Can you work these out from the model? Positions are in its coordinate system, mm. Face numbers are marked on the shaded views. A direction names the side the tool comes from. Coordinates: 2 decimals unless noted, no trailing zeros. Order: outer loops, then holes, each group sorted by start corner. A loop starts at its lowest first (then second) coordinate and runs counter-clockwise, first axis right, second up. Notation, with made-up numbers: (31, -7) -> (40, -7) arc R17 cw to (40, 25) -> close; hole circle Ø6 at (45, -19.5). An arc over 180 degrees is marked (long way). Return JSON: item names as keys, results as strings. Group by question number.
1) If we section it at A-A, the plane y = -1.5: Please give me the cut outline in (x, z), then the cut area to 3 significant figures.
2) If we section it at B-B, the plane z = 7: State how many separate pieces and enclosed holes the cut face has, then the cut area to 3 significant figures.
3) If we section it at C-C, the plane x = -0.25: Please give me the cut outline in (y, z), then the cut area to 3 significant figures.
4) If I drill on probe 1 along Y at (x, z) = (0, 5.75); probe 2 along Y at (x, z) = (-0.25, 4); probe 3 along X at (y, z) = (2.5, 6.5), over which ranges is the centre line in solid material (lowest first)? Write a range as from..to.
5) Thinking about a two-plate mould opening in X: for the marked faces 1, 2 and 3, which applies, +X half, -X half, draft (parallel to the pull), parting line (faces both ways), or undercut?
6) For the marked faces 4 and 5, which set-ups out of +Z, -Z, +X, -X, +Y, -Y let a thin tool reach every point of the face, with its end or its side?
7) If we section it at D-D, the plane x = -1.75: Please give me the cut outline in (y, z).
8) For pin 1 (0.7 mm diameter, centred on y = 7.5, z = 0.5, fed in from +X); pin 2 (1.3 mm diameter, centred on x = 2, z = 3, fed in from -Y); pin 3 (1.3 mm diameter, centred on x = -2, z = 4, fed in from +Y); pin 4 (1.2 mm diameter, centred on x = 0, y = -5.8, fed in from -Z), each with a flat end and sliding along its axis, tell me the tip position at first contact or that it passes through.
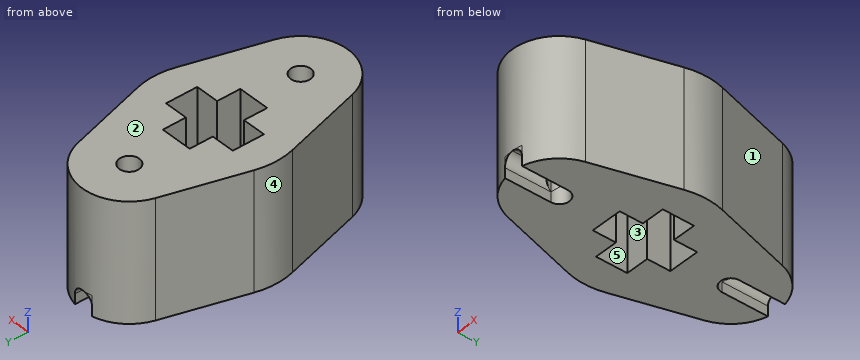
from build123d import *

# Parameters (mm, degrees)
F0_R         = 0.6731
F1_DEPTH     = 7.9375
F3_DEPTH     = 1.3462
F4_T4_DEPTH  = 6.4683311894
F4_S5_R      = 3.175
F4_T6_DEPTH  = 5
F4_S7_R      = 0.6731
F4_T8_DEPTH  = 5
F4_T12_DEPTH = 6.4683311894
F4_S13_R     = 3.175
F4_T14_DEPTH = 5
F4_S15_R     = 0.6731
F4_T16_DEPTH = 5
F4_T20_DEPTH = 6.4683311894
F4_S21_R     = 3.175
F4_T22_DEPTH = 5
F4_S23_R     = 0.6731
F4_T24_DEPTH = 5
F4_T28_DEPTH = 6.4683311894
F4_S29_R     = 3.175
F4_T30_DEPTH = 5
F4_S31_R     = 0.6731
F4_T32_DEPTH = 5


# Not quite as in the source:
# - a fillet or chamfer that OpenCascade refuses, or shapes differently, is made with other operations: its cross-section is extruded or revolved along the edge and cut away or added


with BuildPart() as f1:
    # F0 (on Top) → F1 (new body)
    with BuildSketch(Plane.XY):
        with BuildLine():
            ThreePointArc((-4.5806904159, 1.3033347856), (-4.7625, 0), (-4.5806904159, -1.3033347856))
            Line((-4.5806904159, -1.3033347856), (-3.0537936106, -6.6697545571))
            ThreePointArc((-3.0537936106, -6.6697545571), (0, -8.9758647), (3.0537936106, -6.6697545571))
            Line((3.0537936106, -6.6697545571), (4.5806904159, -1.3033347856))
            ThreePointArc((4.5806904159, -1.3033347856), (4.7625, 0), (4.5806904159, 1.3033347856))
            Line((4.5806904159, 1.3033347856), (3.0537936106, 6.6697545571))
            ThreePointArc((3.0537936106, 6.6697545571), (0, 8.9758647), (-3.0537936106, 6.6697545571))
            Line((-3.0537936106, 6.6697545571), (-4.5806904159, 1.3033347856))
        make_face()
        with Locations((0, -5.8008647)):
            Circle(F0_R, mode=Mode.SUBTRACT)
        Polygon((-1.0574147, 2.6258647), (1.0574147, 2.6258647), (1.0574147, 1.0574147), (2.6258647, 1.0574147), (2.6258647, -1.0574147), (1.0574147, -1.0574147), (1.0574147, -2.6258647), (-1.0574147, -2.6258647), (-1.0574147, -1.0574147), (-2.6258647, -1.0574147), (-2.6258647, 1.0574147), (-1.0574147, 1.0574147), align=None, mode=Mode.SUBTRACT)
        with Locations((0, 5.8008647)):
            Circle(F0_R, mode=Mode.SUBTRACT)
    extrude(amount=F1_DEPTH)

    # F2 (on face) → F3 (cut)
    with BuildSketch(Plane(origin=(0, 0, 0), x_dir=(1, 0, 0), z_dir=(0, 0, -1))):
        with BuildLine():
            Line((-0.6731, 5.8008647), (0.6731, 5.8008647))
            Line((0.6731, 5.8008647), (0.6731, 8.9036958894))
            ThreePointArc((0.6731, 8.9036958894), (0, 8.9758647), (-0.6731, 8.9036958894))
            Line((-0.6731, 8.9036958894), (-0.6731, 5.8008647))
        make_face()
        with BuildLine():
            Line((0.6731, -8.9036958894), (0.6731, -5.8008647))
            Line((0.6731, -5.8008647), (-0.6731, -5.8008647))
            Line((-0.6731, -5.8008647), (-0.6731, -8.9036958894))
            ThreePointArc((-0.6731, -8.9036958894), (0, -8.9758647), (0.6731, -8.9036958894))
        make_face()
    extrude(amount=-F3_DEPTH, mode=Mode.SUBTRACT)

    # F4: fillet of radius 0.6731 on 4 edges, made by hand


with BuildPart() as f4_tool2:
    # F4_s3 → F4_t4 (new body)
    with BuildSketch(Plane.XZ.offset(-10.5864458894)):
        with BuildLine():
            ThreePointArc((0.6731, 0.6731), (0.4759535744, 1.1490535744), (0, 1.3462))
            Line((0, 1.3462), (0.6731, 1.3462))
            Line((0.6731, 1.3462), (0.6731, 0.6731))
        make_face()
    extrude(amount=F4_T4_DEPTH)

    # F4_s5 → F4_t6 (intersect, symmetric)
    with BuildSketch(Plane.XY.offset(1)):
        with Locations((0, 5.8008647)):
            Circle(F4_S5_R)
    extrude(amount=F4_T6_DEPTH, both=True, mode=Mode.INTERSECT)

    # F4_s7 → F4_t8 (cut, symmetric)
    with BuildSketch(Plane.XY.offset(1)):
        with Locations((0, 5.8008647)):
            Circle(F4_S7_R)
    extrude(amount=F4_T8_DEPTH, both=True, mode=Mode.SUBTRACT)


with BuildPart() as f1_1:
    add(f1.part)

    # F4_t1: union F4_tool2
    add(f4_tool2.part)


with BuildPart() as f4_tool10:
    # F4_s11 → F4_t12 (new body)
    with BuildSketch(Plane.XZ.offset(-4.1181147)):
        with BuildLine():
            ThreePointArc((-0.6731, 0.6731), (-0.4759535744, 1.1490535744), (0, 1.3462))
            Line((0, 1.3462), (-0.6731, 1.3462))
            Line((-0.6731, 1.3462), (-0.6731, 0.6731))
        make_face()
    extrude(amount=-F4_T12_DEPTH)

    # F4_s13 → F4_t14 (intersect, symmetric)
    with BuildSketch(Plane.XY.offset(1)):
        with Locations((0, 5.8008647)):
            Circle(F4_S13_R)
    extrude(amount=F4_T14_DEPTH, both=True, mode=Mode.INTERSECT)

    # F4_s15 → F4_t16 (cut, symmetric)
    with BuildSketch(Plane.XY.offset(1)):
        with Locations((0, 5.8008647)):
            Circle(F4_S15_R)
    extrude(amount=F4_T16_DEPTH, both=True, mode=Mode.SUBTRACT)


with BuildPart() as f1_2:
    add(f1_1.part)

    # F4_t9: union F4_tool10
    add(f4_tool10.part)


with BuildPart() as f4_tool18:
    # F4_s19 → F4_t20 (new body)
    with BuildSketch(Plane.XZ.offset(4.1181147)):
        with BuildLine():
            ThreePointArc((0.6731, 0.6731), (0.4759535744, 1.1490535744), (0, 1.3462))
            Line((0, 1.3462), (0.6731, 1.3462))
            Line((0.6731, 1.3462), (0.6731, 0.6731))
        make_face()
    extrude(amount=F4_T20_DEPTH)

    # F4_s21 → F4_t22 (intersect, symmetric)
    with BuildSketch(Plane.XY.offset(1)):
        with Locations((0, -5.8008647)):
            Circle(F4_S21_R)
    extrude(amount=F4_T22_DEPTH, both=True, mode=Mode.INTERSECT)

    # F4_s23 → F4_t24 (cut, symmetric)
    with BuildSketch(Plane.XY.offset(1)):
        with Locations((0, -5.8008647)):
            Circle(F4_S23_R)
    extrude(amount=F4_T24_DEPTH, both=True, mode=Mode.SUBTRACT)


with BuildPart() as f1_3:
    add(f1_2.part)

    # F4_t17: union F4_tool18
    add(f4_tool18.part)


with BuildPart() as f4_tool26:
    # F4_s27 → F4_t28 (new body)
    with BuildSketch(Plane.XZ.offset(10.5864458894)):
        with BuildLine():
            ThreePointArc((-0.6731, 0.6731), (-0.4759535744, 1.1490535744), (0, 1.3462))
            Line((0, 1.3462), (-0.6731, 1.3462))
            Line((-0.6731, 1.3462), (-0.6731, 0.6731))
        make_face()
    extrude(amount=-F4_T28_DEPTH)

    # F4_s29 → F4_t30 (intersect, symmetric)
    with BuildSketch(Plane.XY.offset(1)):
        with Locations((0, -5.8008647)):
            Circle(F4_S29_R)
    extrude(amount=F4_T30_DEPTH, both=True, mode=Mode.INTERSECT)

    # F4_s31 → F4_t32 (cut, symmetric)
    with BuildSketch(Plane.XY.offset(1)):
        with Locations((0, -5.8008647)):
            Circle(F4_S31_R)
    extrude(amount=F4_T32_DEPTH, both=True, mode=Mode.SUBTRACT)


with BuildPart() as f1_4:
    add(f1_3.part)

    # F4_t25: union F4_tool26
    add(f4_tool26.part)


solid = f1_4.part
Result sheet:
{
 "1": {"outline": "(-4.52, 0) -> (-1.06, 0) -> (-1.06, 7.94) -> (-4.52, 7.94) -> close; (1.06, 0) -> (4.52, 0) -> (4.52, 7.94) -> (1.06, 7.94) -> close", "area": "55.0 mm2"},
 "2": {"separate pieces": "1", "enclosed holes": "3", "area": "107 mm2"},
 "3": {"outline": "(-8.97, 1.3) -> (-6.43, 1.3) -> (-6.43, 7.94) -> (-8.97, 7.94) -> close; (-5.18, 0) -> (-2.63, 0) -> (-2.63, 7.94) -> (-5.18, 7.94) -> close; (2.63, 0) -> (5.18, 0) -> (5.18, 7.94) -> (2.63, 7.94) -> close; (6.43, 1.3) -> (8.97, 1.3) -> (8.97, 7.94) -> (6.43, 7.94) -> close", "area": "74.2 mm2"},
 "4": {"probe 1": "y = -8.98..-6.47, -5.13..-2.63, 2.63..5.13, 6.47..8.98", "probe 2": "y = -8.97..-6.43, -5.18..-2.63, 2.63..5.18, 6.43..8.97", "probe 3": "x = -4.24..-1.06, 1.06..4.24"},
 "5": {"face 1": "+X half", "face 2": "draft", "face 3": "undercut"},
 "6": {"face 4": "+Z, -Z, -X", "face 5": "+Z, -Z"},
 "7": {"outline": "(-8.45, 0) -> (-1.06, 0) -> (-1.06, 7.94) -> (-8.45, 7.94) -> close; (1.06, 0) -> (8.45, 0) -> (8.45, 7.94) -> (1.06, 7.94) -> close"},
 "8": {"pin 1": "stops at x = 2.87", "pin 2": "stops at y = -8.67", "pin 3": "stops at y = 8.67", "pin 4": "passes through"}
}
